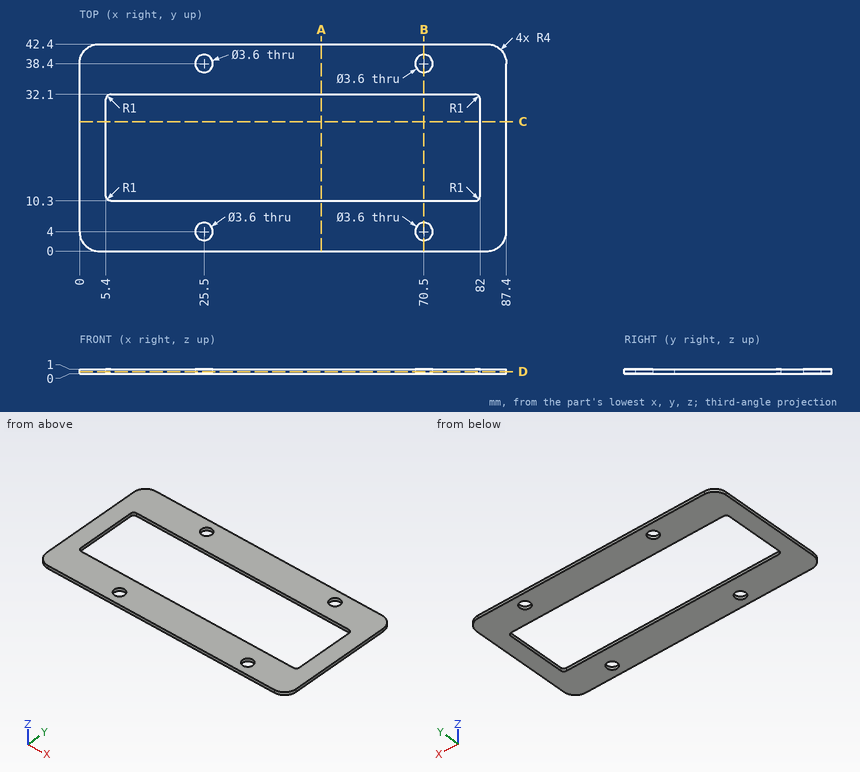
Answer from the drawing. Dimensions are ordinates in mm from the lowest x, y and z of the part. Coordinates: 2 decimals unless noted, no trailing zeros. Write each loop counter-clockwise with the first axis right and the second up, starting at its lowest first coordinate (ties: lowest second). Pieces come first, ordered by that corner, then holes. Notation, with made-up numbers: M 9.25,56 L 64.25,56 A12 cw 64.25,70 Z; hole C 31,57 d10. An arc over 180 degrees is marked long. Use one line per item in the form item = value. Start each with the question number.
1. The part is cut by section A-A (x = 49.5). Give the vertices of the cut face in (y, z).
2. The part is cut by section C-C (y = 26.5). Give the vertices of the cut face in (x, z), plus the area to 3 significant figures.
3. The part is cut by section B-B (x = 70.5). Give the vertices of the cut face in (y, z).
4. Straight lines are drawn through the part: probe 1 along Y at (x, z) = (70.5, 0.2); probe 2 along X at (y, z) = (13.5, 0.7); probe 3 along Y at (x, z) = (8.5, 0.4). For each, find the intervals that lie inside material, in ascending order. Write a range as from..to.
5. The part is cut by section D-D (z = 0.5). Give the vertices of the cut face in (x, y).
Evaluation:
q1.outline = M 0,0 L 10.3,0 L 10.3,1 L 0,1 Z; M 32.1,0 L 42.4,0 L 42.4,1 L 32.1,1 Z
q2.outline = M 0,0 L 5.4,0 L 5.4,1 L 0,1 Z; M 82,0 L 87.4,0 L 87.4,1 L 82,1 Z
q2.area = 10.8 mm^2
q3.outline = M 0,0 L 2.2,0 L 2.2,1 L 0,1 Z; M 5.8,0 L 10.3,0 L 10.3,1 L 5.8,1 Z; M 32.1,0 L 36.6,0 L 36.6,1 L 32.1,1 Z; M 40.2,0 L 42.4,0 L 42.4,1 L 40.2,1 Z
q4.probe_1 = 0..2.2, 5.8..10.3, 32.1..36.6, 40.2..42.4
q4.probe_2 = 0..5.4, 82..87.4
q4.probe_3 = 0..10.3, 32.1..42.4
q5.outline = M 0,4 A4 ccw 4,0 L 83.4,0 A4 ccw 87.4,4 L 87.4,38.4 A4 ccw 83.4,42.4 L 4,42.4 A4 ccw 0,38.4 Z; hole M 5.4,11.3 A1 ccw 6.4,10.3 L 81,10.3 A1 ccw 82,11.3 L 82,31.1 A1 ccw 81,32.1 L 6.4,32.1 A1 ccw 5.4,31.1 Z; hole C 25.5,4 d3.6; hole C 25.5,38.4 d3.6; hole C 70.5,4 d3.6; hole C 70.5,38.4 d3.6
